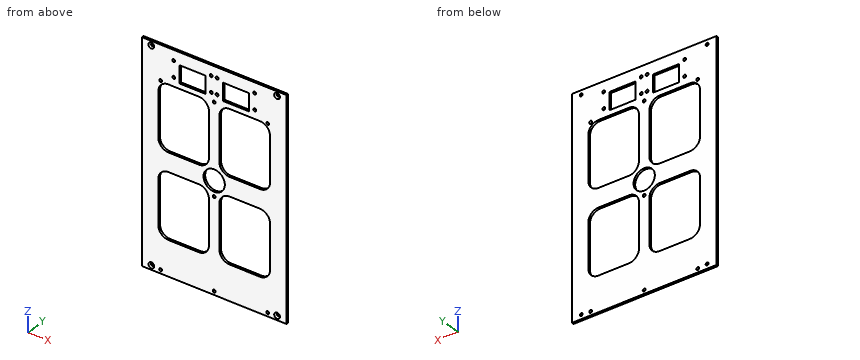
from build123d import *

# Parameters (mm, degrees)
F0_W           = 100
F0_H           = 150
F0_R           = 7.3677826157
F1_DEPTH       = 1.5
F3_D           = 2
F3_CSINK_D     = 4
F3_CSINK_ANGLE = 90
F4_D           = 2
F6_D           = 2


# Not quite as in the source:
# - a feature names something its author has since deleted; it is built from what else it names


with BuildPart() as f1:
    # F0 (on Front) → F1 (new body)
    with BuildSketch(Plane.XZ):
        Rectangle(F0_W, F0_H)
        with BuildLine():
            Line((-31.6183936375, -6.4180564158), (-10.6183936375, -6.4180564158))
            ThreePointArc((-10.6183936375, -6.4180564158), (-5.6686461691, -8.4683089475), (-3.6183936375, -13.4180564158))
            Line((-3.6183936375, -13.4180564158), (-3.6183936375, -44))
            ThreePointArc((-3.6183936375, -44), (-5.6686461691, -48.9497474683), (-10.6183936375, -51))
            Line((-10.6183936375, -51), (-31.6183936375, -51))
            ThreePointArc((-31.6183936375, -51), (-36.5681411058, -48.9497474683), (-38.6183936375, -44))
            Line((-38.6183936375, -44), (-38.6183936375, -13.4180564158))
            ThreePointArc((-38.6183936375, -13.4180564158), (-36.5681411058, -8.4683089475), (-31.6183936375, -6.4180564158))
        make_face(mode=Mode.SUBTRACT)
        with BuildLine():
            ThreePointArc((38.6183936375, -44), (36.5681411058, -48.9497474683), (31.6183936375, -51))
            Line((31.6183936375, -51), (10.6183936375, -51))
            ThreePointArc((10.6183936375, -51), (5.6686461691, -48.9497474683), (3.6183936375, -44))
            Line((3.6183936375, -44), (3.6183936375, -13.4180564158))
            ThreePointArc((3.6183936375, -13.4180564158), (5.6686461691, -8.4683089475), (10.6183936375, -6.4180564158))
            Line((10.6183936375, -6.4180564158), (31.6183936375, -6.4180564158))
            ThreePointArc((31.6183936375, -6.4180564158), (36.5681411058, -8.4683089475), (38.6183936375, -13.4180564158))
            Line((38.6183936375, -13.4180564158), (38.6183936375, -44))
        make_face(mode=Mode.SUBTRACT)
        with BuildLine():
            ThreePointArc((-3.6183936375, 13.4180564158), (-5.6686461691, 8.4683089475), (-10.6183936375, 6.4180564158))
            Line((-10.6183936375, 6.4180564158), (-31.6183936375, 6.4180564158))
            ThreePointArc((-31.6183936375, 6.4180564158), (-36.5681411058, 8.4683089475), (-38.6183936375, 13.4180564158))
            Line((-38.6183936375, 13.4180564158), (-38.6183936375, 44))
            ThreePointArc((-38.6183936375, 44), (-36.5681411058, 48.9497474683), (-31.6183936375, 51))
            Line((-31.6183936375, 51), (-10.6183936375, 51))
            ThreePointArc((-10.6183936375, 51), (-5.6686461691, 48.9497474683), (-3.6183936375, 44))
            Line((-3.6183936375, 44), (-3.6183936375, 13.4180564158))
        make_face(mode=Mode.SUBTRACT)
        Polygon((-24, 54.5), (-24, 66.5), (-15, 66.5), (-6, 66.5), (-6, 54.5), (-15, 54.5), align=None, mode=Mode.SUBTRACT)
        Circle(F0_R, mode=Mode.SUBTRACT)
        with BuildLine():
            ThreePointArc((10.6183936375, 6.4180564158), (5.6686461691, 8.4683089475), (3.6183936375, 13.4180564158))
            Line((3.6183936375, 13.4180564158), (3.6183936375, 44))
            ThreePointArc((3.6183936375, 44), (5.6686461691, 48.9497474683), (10.6183936375, 51))
            Line((10.6183936375, 51), (31.6183936375, 51))
            ThreePointArc((31.6183936375, 51), (36.5681411058, 48.9497474683), (38.6183936375, 44))
            Line((38.6183936375, 44), (38.6183936375, 13.4180564158))
            ThreePointArc((38.6183936375, 13.4180564158), (36.5681411058, 8.4683089475), (31.6183936375, 6.4180564158))
            Line((31.6183936375, 6.4180564158), (10.6183936375, 6.4180564158))
        make_face(mode=Mode.SUBTRACT)
        Polygon((6, 54.5), (6, 66.5), (15, 66.5), (24, 66.5), (24, 54.5), (15, 54.5), align=None, mode=Mode.SUBTRACT)
    extrude(amount=F1_DEPTH)

    # F3 (through all)
    with Locations(Plane.XZ.offset(1.5)):
        with Locations((-43.5, -72), (43.5, -72), (43.5, 72), (-43.5, 72)):
            CounterSinkHole(F3_D / 2, F3_CSINK_D / 2, counter_sink_angle=F3_CSINK_ANGLE)

    # F4 (through all)
    with Locations(Plane(origin=(0, 0, 0), x_dir=(1, 0, 0), z_dir=(0, 1, 0))):
        with Locations((-28, -68), (-28, -57), (-2, -57), (-2, -68), (2, -68), (2, -57), (28, -57), (28, -68)):
            Hole(F4_D / 2)

    # F6 (through all)
    with Locations(Plane(origin=(0, 0, 0), x_dir=(1, 0, 0), z_dir=(0, 1, 0))):
        with Locations((-37, 72.5), (0, 72.5), (37, 72.5), (0, 10.5), (0, -51.5), (37, -51.5), (-37, -51.5)):
            Hole(F6_D / 2)


solid = f1.part
Geometry: final body of the model. Coordinates: model frame, mm. Coordinates: 2 decimals unless noted, no trailing zeros. Order: outer loops, then holes, each group sorted by start corner. A loop starts at its lowest first (then second) coordinate and runs counter-clockwise, first axis right, second up. Notation, with made-up numbers: (14, 45.5) - (32, 45.5) arc R24 cw to (32, 75.5) - close; hole circle Ø7 at (60, -4.5). An arc over 180 degrees is marked (long way). Use one line per item in the form item = value.
1) Pin query (flat end, axial travel): pin 1 (1.6 mm diameter, centred on x = 37, z = 51.5, fed in from -Y); pin 2 (2.5 mm diameter, centred on x = -28, z = 68, fed in from +Y). Return the tip coordinate at first contact, or that it passes through.
Solutions:
pin_1 = through
pin_2 = 0
2) Section A-A (x = 16). Return loops of the section in (y, z), then the cut area to 3 significant figures.
Solutions:
outline = (-1.5, -75) - (0, -75) - (0, -51) - (-1.5, -51) - close; (-1.5, -6.42) - (0, -6.42) - (0, 6.42) - (-1.5, 6.42) - close; (-1.5, 51) - (0, 51) - (0, 54.5) - (-1.5, 54.5) - close; (-1.5, 66.5) - (0, 66.5) - (0, 75) - (-1.5, 75) - close
area = 73.3 mm^2
3) Section B-B (z = -17). Return loops of the section in (x, y).
Solutions:
outline = (-50, -1.5) - (-38.62, -1.5) - (-38.62, 0) - (-50, 0) - close; (-3.62, -1.5) - (3.62, -1.5) - (3.62, 0) - (-3.62, 0) - close; (38.62, -1.5) - (50, -1.5) - (50, 0) - (38.62, 0) - close
4) Ray query, L1, parallel to X at y = -0.15, z = -42; L2, parallel to Z at x = 15, y = -0.7; L3, parallel to Z at x = -28, y = -1.2. Return the intervals inside material, ascending.
Solutions:
L1 = -50 to -38.62, -3.62 to 3.62, 38.62 to 50
L2 = -75 to -51, -6.42 to 6.42, 51 to 54.5, 66.5 to 75
L3 = -75 to -51, -6.42 to 6.42, 51 to 56, 58 to 67, 69 to 75
